Could you check a few things on this model? Use its own coordinates, in mm. Give positions to 0.01 mm unless a question says otherwise; leave off trailing zeros. Write each loop counter-clockwise with the first axis right and the second up, starting at its lowest first coordinate (ties: lowest second). Pieces come first, ordered by that corner, then holes. Notation, with made-up numbers: M 22.25,17 L 41.25,17 A18 cw 41.25,23 Z; hole C 24,79.5 d8. An arc over 180 degrees is marked long. Use one line per item in the form item = value.
from build123d import *

# Parameters (mm, degrees)
F0_R     = 16.5
F1_DEPTH = 3
F2_DEPTH = 3


with BuildPart() as f1:
    # F0 (on Front) → F1 (new body)
    with BuildSketch(Plane.XZ):
        with BuildLine():
            ThreePointArc((10.650584, 4.982898), (7.88696, 6.201296), (4.998663, 7.084391))
            ThreePointArc((4.998663, 7.084391), (4.999666, 7.142192), (5, 7.2))
            Line((5, 7.2), (2.811259, 14.245932))
            Line((2.811259, 14.245932), (-2.811259, 14.245932))
            Line((-2.811259, 14.245932), (-4.907152, 7.498892))
            ThreePointArc((-4.907152, 7.498892), (-7.859128, 6.860178), (-10.714879, 5.876919))
            ThreePointArc((-10.714879, 5.876919), (-10.748042, 5.92427), (-10.781751, 5.971235))
            Line((-10.781751, 5.971235), (-16.693975, 10.385003))
            Line((-16.693975, 10.385003), (-21.242687, 7.080171))
            Line((-21.242687, 7.080171), (-18.97249, 0.389765))
            ThreePointArc((-18.97249, 0.389765), (-20.985262, -1.862092), (-22.717668, -4.336134))
            ThreePointArc((-22.717668, -4.336134), (-22.77233, -4.317319), (-22.827205, -4.299138))
            Line((-22.827205, -4.299138), (-30.204643, -4.203442))
            Line((-30.204643, -4.203442), (-31.942096, -9.550773))
            Line((-31.942096, -9.550773), (-26.172947, -13.629037))
            ThreePointArc((-26.172947, -13.629037), (-26.477705, -16.633906), (-26.425045, -19.65373))
            ThreePointArc((-26.425045, -19.65373), (-26.480327, -19.670638), (-26.535409, -19.688184))
            Line((-26.535409, -19.688184), (-32.56013, -23.947114))
            Line((-32.56013, -23.947114), (-30.822677, -29.294445))
            Line((-30.822677, -29.294445), (-23.758194, -29.202809))
            ThreePointArc((-23.758194, -29.202809), (-22.238531, -31.812931), (-20.42092, -34.225068))
            ThreePointArc((-20.42092, -34.225068), (-20.455705, -34.27124), (-20.489955, -34.317812))
            Line((-20.489955, -34.317812), (-22.860721, -41.3046))
            Line((-22.860721, -41.3046), (-18.312009, -44.609433))
            Line((-18.312009, -44.609433), (-12.650584, -40.382898))
            ThreePointArc((-12.650584, -40.382898), (-9.88696, -41.601296), (-6.998663, -42.484391))
            ThreePointArc((-6.998663, -42.484391), (-6.999666, -42.542192), (-7, -42.6))
            Line((-7, -42.6), (-4.811259, -49.645932))
            Line((-4.811259, -49.645932), (0.811259, -49.645932))
            Line((0.811259, -49.645932), (2.907152, -42.898892))
            ThreePointArc((2.907152, -42.898892), (5.859128, -42.260178), (8.714879, -41.276919))
            ThreePointArc((8.714879, -41.276919), (8.748042, -41.32427), (8.781751, -41.371235))
            Line((8.781751, -41.371235), (14.693975, -45.785003))
            Line((14.693975, -45.785003), (19.242687, -42.480171))
            Line((19.242687, -42.480171), (16.97249, -35.789765))
            ThreePointArc((16.97249, -35.789765), (18.985262, -33.537908), (20.717668, -31.063866))
            ThreePointArc((20.717668, -31.063866), (20.77233, -31.082681), (20.827205, -31.100862))
            Line((20.827205, -31.100862), (28.204643, -31.196558))
            Line((28.204643, -31.196558), (29.942096, -25.849227))
            Line((29.942096, -25.849227), (24.172947, -21.770963))
            ThreePointArc((24.172947, -21.770963), (24.477705, -18.766094), (24.425045, -15.74627))
            ThreePointArc((24.425045, -15.74627), (24.480327, -15.729362), (24.535409, -15.711816))
            Line((24.535409, -15.711816), (30.56013, -11.452886))
            Line((30.56013, -11.452886), (28.822677, -6.105555))
            Line((28.822677, -6.105555), (21.758194, -6.197191))
            ThreePointArc((21.758194, -6.197191), (20.238531, -3.587069), (18.42092, -1.174932))
            ThreePointArc((18.42092, -1.174932), (18.455705, -1.12876), (18.489955, -1.082188))
            Line((18.489955, -1.082188), (20.860721, 5.9046))
            Line((20.860721, 5.9046), (16.312009, 9.209433))
            Line((16.312009, 9.209433), (10.650584, 4.982898))
        make_face()
        with Locations((-1, -17.7)):
            Circle(F0_R, mode=Mode.SUBTRACT)
    extrude(amount=F1_DEPTH)

    # F0 (on Front) → F2 (join)
    with BuildSketch(Plane.XZ):
        with BuildLine():
            ThreePointArc((10.650584, 4.982898), (7.88696, 6.201296), (4.998663, 7.084391))
            ThreePointArc((4.998663, 7.084391), (4.999666, 7.142192), (5, 7.2))
            Line((5, 7.2), (2.811259, 14.245932))
            Line((2.811259, 14.245932), (-2.811259, 14.245932))
            Line((-2.811259, 14.245932), (-4.907152, 7.498892))
            ThreePointArc((-4.907152, 7.498892), (-7.859128, 6.860178), (-10.714879, 5.876919))
            ThreePointArc((-10.714879, 5.876919), (-10.748042, 5.92427), (-10.781751, 5.971235))
            Line((-10.781751, 5.971235), (-16.693975, 10.385003))
            Line((-16.693975, 10.385003), (-21.242687, 7.080171))
            Line((-21.242687, 7.080171), (-18.97249, 0.389765))
            ThreePointArc((-18.97249, 0.389765), (-20.985262, -1.862092), (-22.717668, -4.336134))
            ThreePointArc((-22.717668, -4.336134), (-22.77233, -4.317319), (-22.827205, -4.299138))
            Line((-22.827205, -4.299138), (-30.204643, -4.203442))
            Line((-30.204643, -4.203442), (-31.942096, -9.550773))
            Line((-31.942096, -9.550773), (-26.172947, -13.629037))
            ThreePointArc((-26.172947, -13.629037), (-26.477705, -16.633906), (-26.425045, -19.65373))
            ThreePointArc((-26.425045, -19.65373), (-26.480327, -19.670638), (-26.535409, -19.688184))
            Line((-26.535409, -19.688184), (-32.56013, -23.947114))
            Line((-32.56013, -23.947114), (-30.822677, -29.294445))
            Line((-30.822677, -29.294445), (-23.758194, -29.202809))
            ThreePointArc((-23.758194, -29.202809), (-22.238531, -31.812931), (-20.42092, -34.225068))
            ThreePointArc((-20.42092, -34.225068), (-20.455705, -34.27124), (-20.489955, -34.317812))
            Line((-20.489955, -34.317812), (-22.860721, -41.3046))
            Line((-22.860721, -41.3046), (-18.312009, -44.609433))
            Line((-18.312009, -44.609433), (-12.650584, -40.382898))
            ThreePointArc((-12.650584, -40.382898), (-9.88696, -41.601296), (-6.998663, -42.484391))
            ThreePointArc((-6.998663, -42.484391), (-6.999666, -42.542192), (-7, -42.6))
            Line((-7, -42.6), (-4.811259, -49.645932))
            Line((-4.811259, -49.645932), (0.811259, -49.645932))
            Line((0.811259, -49.645932), (2.907152, -42.898892))
            ThreePointArc((2.907152, -42.898892), (5.859128, -42.260178), (8.714879, -41.276919))
            ThreePointArc((8.714879, -41.276919), (8.748042, -41.32427), (8.781751, -41.371235))
            Line((8.781751, -41.371235), (14.693975, -45.785003))
            Line((14.693975, -45.785003), (19.242687, -42.480171))
            Line((19.242687, -42.480171), (16.97249, -35.789765))
            ThreePointArc((16.97249, -35.789765), (18.985262, -33.537908), (20.717668, -31.063866))
            ThreePointArc((20.717668, -31.063866), (20.77233, -31.082681), (20.827205, -31.100862))
            Line((20.827205, -31.100862), (28.204643, -31.196558))
            Line((28.204643, -31.196558), (29.942096, -25.849227))
            Line((29.942096, -25.849227), (24.172947, -21.770963))
            ThreePointArc((24.172947, -21.770963), (24.477705, -18.766094), (24.425045, -15.74627))
            ThreePointArc((24.425045, -15.74627), (24.480327, -15.729362), (24.535409, -15.711816))
            Line((24.535409, -15.711816), (30.56013, -11.452886))
            Line((30.56013, -11.452886), (28.822677, -6.105555))
            Line((28.822677, -6.105555), (21.758194, -6.197191))
            ThreePointArc((21.758194, -6.197191), (20.238531, -3.587069), (18.42092, -1.174932))
            ThreePointArc((18.42092, -1.174932), (18.455705, -1.12876), (18.489955, -1.082188))
            Line((18.489955, -1.082188), (20.860721, 5.9046))
            Line((20.860721, 5.9046), (16.312009, 9.209433))
            Line((16.312009, 9.209433), (10.650584, 4.982898))
        make_face()
        with Locations((-1, -17.7)):
            Circle(F0_R, mode=Mode.SUBTRACT)
    extrude(amount=F2_DEPTH)


solid = f1.part
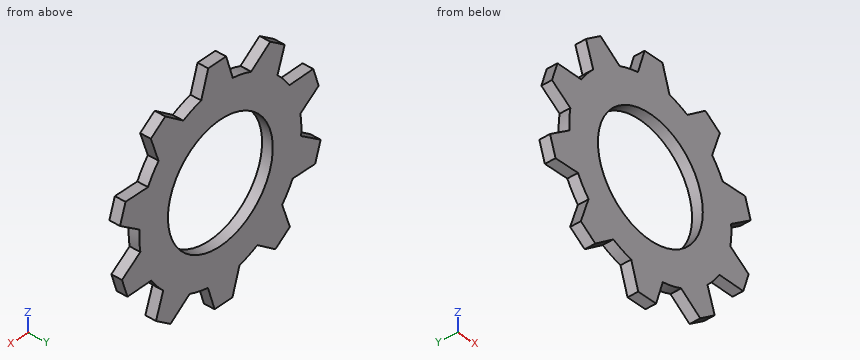
1) I want a section at A-A, the plane x = -1. Please give me the cut outline in (y, z).
Checked values:
outline = M -3,-49.65 L 0,-49.65 L 0,-34.2 L -3,-34.2 Z; M -3,-1.2 L 0,-1.2 L 0,14.25 L -3,14.25 Z
2) If I drill on L1, parallel to Z at x = -1, y = -2.2; L2, parallel to X at y = -0.65, z = -2.5; L3, parallel to Z at x = 26.5, y = -2.4, over which ranges is the centre line in solid material (lowest first)?
Checked values:
L1 = -49.65 to -34.2, -1.2 to 14.25
L2 = -21.47 to -7.42, 5.42 to 19.47
L3 = -31.17 to -23.42, -14.32 to -6.14
3) For pin 1 Ø1.5 at (y, z) = (-2.5, -1.5) entering from -X, with a flat end and sliding along its axis, tell me the tip position at first contact or that it passes through.
Checked values:
pin_1 = -21.29
4) I want a section at B-B, the plane z = -17.7. Please give me the cut outline in (x, y), plus the area to 3 significant figures.
Checked values:
outline = M -26.5,-3 L -17.5,-3 L -17.5,0 L -26.5,0 Z; M 15.5,-3 L 24.5,-3 L 24.5,0 L 15.5,0 Z
area = 54.0 mm2
